The figure shows three views and two pictorial views of one solid part (mm, origin at its lowest corner). Answer the questions. Round coordinates to 2 decimals unless told otherwise and drop trailing zeros. Write each loop counter-clockwise with the first axis right and the second up, starting at its lowest first coordinate (ties: lowest second). Pieces come first, ordered by that corner, then holes. Notation, with made-up numbers: M 71,58.25 L 75,58.25 A19 ccw 75,84.25 Z; hole C 56.5,-3.5 d8. An arc over 180 degrees is marked long. Answer in a Markdown table with one row per item.
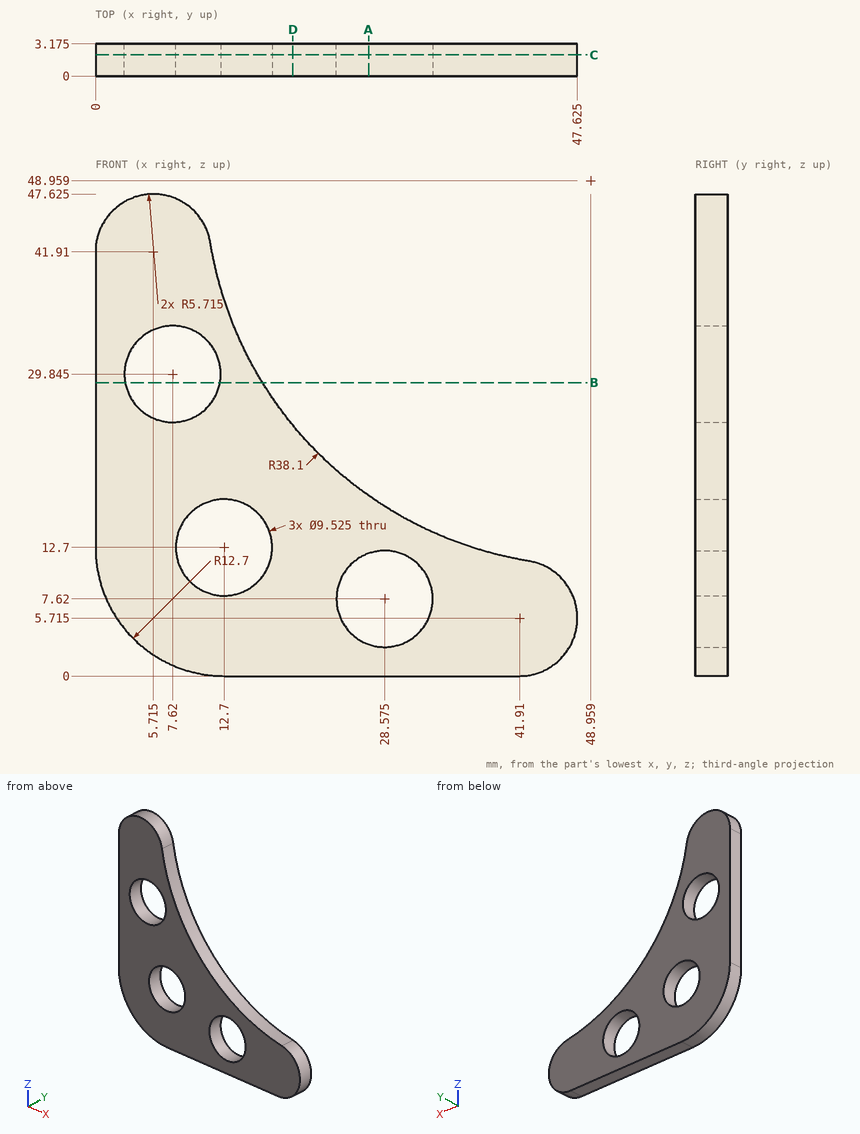
1. The part is cut by section D-D (x = 19.5). Determine the outline of the cut face in (y, z) (3 decimals).
Calculated:
| item | result |
|---|---|
| outline | M 0,0 L 3.175,0 L 3.175,24.798 L 0,24.798 Z |
2. The part is cut by section A-A (x = 27). Determine the outline of the cut face in (y, z) (1 decimal).
Calculated:
| item | result |
|---|---|
| outline | M 0,0 L 3.2,0 L 3.2,3.1 L 0,3.1 Z; M 0,12.1 L 3.2,12.1 L 3.2,17.8 L 0,17.8 Z |
3. Given pin 1 (7.5 mm diameter, centred on x = 7.62, z = 29.845, fed in from +Y); pin 2 (12.5 mm diameter, centred on x = 28.575, z = 7.62, fed in from -Y); pin 3 (1.5 mm diameter, centred on x = 32.5, y = 2.5, fed in from +Z), each flat-ended and moving along its own axis, determine where each tip first touches the part or whether it passes through.
Calculated:
| item | result |
|---|---|
| pin 1 | passes through |
| pin 2 | stops at y = 0 |
| pin 3 | stops at z = 14.97 |
4. The part is cut by section C-C (y = 2.1). Determine the outline of the cut face in (x, z) (1 decimal), plus the area to 3 significant figures.
Calculated:
| item | result |
|---|---|
| outline | M 0,12.7 A12.7 ccw 12.7,0 L 41.9,0 A5.7 ccw 42.8,11.4 A38.1 cw 11.4,42.8 A5.7 ccw 0,41.9 Z; hole C 7.6,29.8 d9.5; hole C 12.7,12.7 d9.5; hole C 28.6,7.6 d9.5 |
| area | 955 mm² |
5. Consider line 1 along Z through (x, y) = (30.5, 1.15); line 2 along Z through (x, y) = (29.5, 1.15); line 3 along X through (y, z) = (2, 27) (1 decimal). Determine where each line is inside the solid, lowest interval first. Write a range as from..to.
Calculated:
| item | result |
|---|---|
| line 1 | z = 0..3.26, 11.98..15.63 |
| line 2 | z = 0..2.95, 12.29..16.2 |
| line 3 | x = 0..3.8, 11.4..17.8 |
6. The part is cut by section B-B (z = 29). Determine the outline of the cut face in (x, y) (1 decimal).
Calculated:
| item | result |
|---|---|
| outline | M 0,0 L 2.9,0 L 2.9,3.2 L 0,3.2 Z; M 12.3,0 L 16.5,0 L 16.5,3.2 L 12.3,3.2 Z |
